The figure shows three views and two pictorial views of one solid part (mm, origin at its lowest corner). Answer the questions. A direction names the side the tool comes from. Coordinates: 2 decimals unless noted, no trailing zeros. Loops run counter-clockwise (first coordinate to the right, second up) from the corner with the lowest first, then second, coordinate; pieces in that order, holes last.
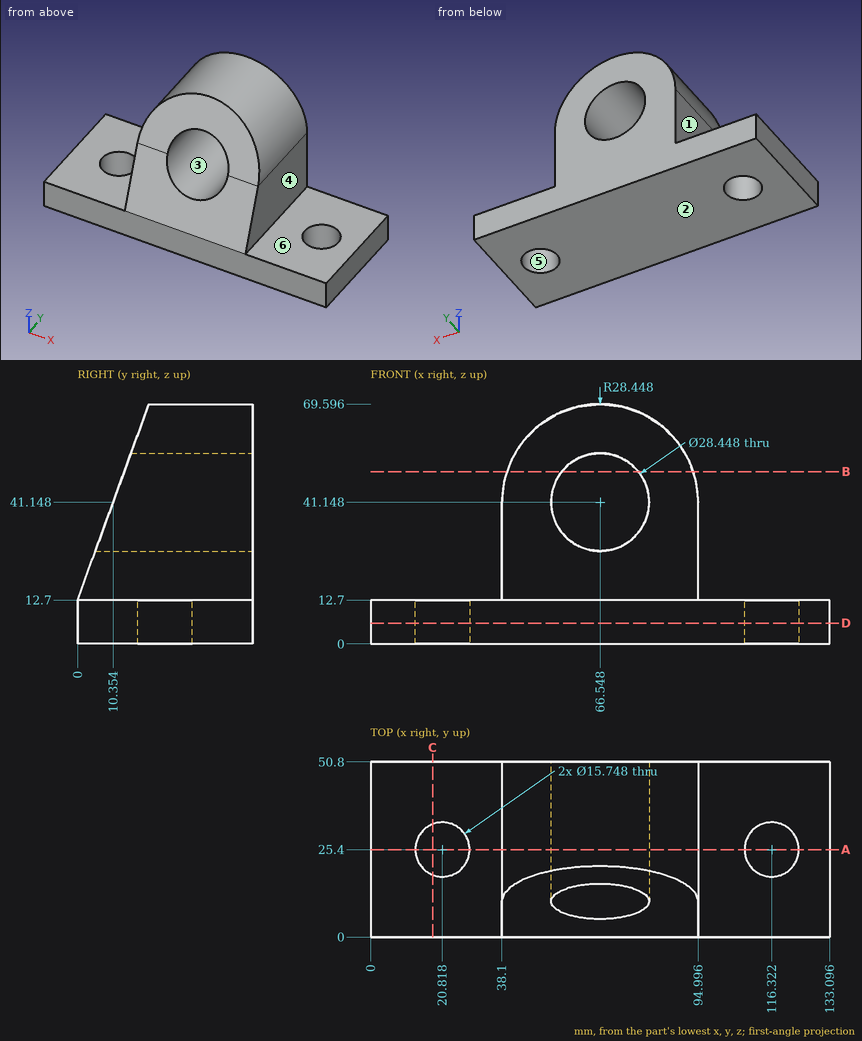
1. A cutting plane is placed at A-A, the plane y = 25.4. Give the vertices of the cut face in (x, z) (1 decimal).
2. A cutting plane is placed at D-D, the plane z = 6. Give the vertices of the cut face in (x, y), then the cut area to 3 significant figures.
3. Each of these flat-tipped pins is pushed along its axis until it touches: P1, Ø10, axis at y = 20, z = 42.5, coming from the -X side; P2, Ø12, axis at x = 93.5, y = 22, coming from the +Z side; P3, Ø3, axis at x = 50.5, z = 57, coming from the -Y side. Where does it stop, or does it pass through?
4. For the marked faces 1 and 2, determine the directions among +Z, -Z, +X, -X, +Y, -Y from which every point of the face is accessible in a straight line to the end or side of a thin tool.
5. Straight lines are drawn through the part: probe 1 along X at (y, z) = (25, 8) (1 decimal); probe 2 along Z at (x, y) = (29, 31.5); probe 3 along X at (y, z) = (29.5, 31) (1 decimal). For each, find the intervals that lie inside material, in ascending order.
6. A cutting plane is placed at C-C, the plane x = 18. Give the vertices of the cut face in (y, z).
7. Determine the mould class of the marked faces 3, 4, 5 and 6 for opening direction X: released by +X, released by -X, zero draft, split by the parting line, or undercut.
8. A cutting plane is placed at B-B, the plane z = 50. Give the vertices of the cut face in (x, y) (1 decimal), then the cut area to 3 significant figures.
Answers below:
1. outline: (0, 0) - (12.9, 0) - (12.9, 12.7) - (0, 12.7) - close; (28.7, 0) - (108.4, 0) - (108.4, 12.7) - (95, 12.7) - (95, 41.1) arc R28.4 ccw to (38.1, 41.1) - (38.1, 12.7) - (28.7, 12.7) - close; (124.2, 0) - (133.1, 0) - (133.1, 12.7) - (124.2, 12.7) - close; hole circle Ø28.4 at (66.5, 41.1)
2. outline: (0, 0) - (133.1, 0) - (133.1, 50.8) - (0, 50.8) - close; hole circle Ø15.75 at (20.82, 25.4); hole circle Ø15.75 at (116.32, 25.4)
2. area: 6,370 mm2
3. P1: stops at x = 38.1
3. P2: stops at z = 60.39
3. P3: stops at y = 15.58
4. face 1: +Z, -X, +Y, -Y
4. face 2: -Z, +X, -X, +Y, -Y
5. probe 1: x = 0 to 13, 28.7 to 108.5, 124.2 to 133.1
5. probe 2: z = 0 to 12.7
5. probe 3: x = 38.1 to 56.6, 76.5 to 95
6. outline: (0, 0) - (18.05, 0) - (18.05, 12.7) - (0, 12.7) - close; (32.75, 0) - (50.8, 0) - (50.8, 12.7) - (32.75, 12.7) - close
7. face 3: undercut
7. face 4: released by +X
7. face 5: undercut
7. face 6: zero draft
8. outline: (39.5, 13.6) - (55.4, 13.6) - (55.4, 50.8) - (39.5, 50.8) - close; (77.7, 13.6) - (93.6, 13.6) - (93.6, 50.8) - (77.7, 50.8) - close
8. area: 1,180 mm2
